Can you work these out from the model? Positions are in its coordinate system, mm. A direction names the side the tool comes from. Coordinates: 2 decimals unless noted, no trailing zeros. Order: outer loops, then holes, each group sorted by start corner. A loop starts at its lowest first (then second) coordinate and runs counter-clockwise, first axis right, second up. Notation, with made-up numbers: (14, -1.75) - (57, -1.75) arc R24 ccw to (57, 21.25) - close; hole circle Ø10 at (1, 24.5). An arc over 180 degrees is marked (long way). Return JSON: item names as keys, results as strings. Group by question number.
1) If I drill on line 1 along Z through (x, y) = (3.75, -1); line 2 along Z through (x, y) = (8.75, 1.75); line 3 along X through (y, z) = (-1.5, -2.25), over which ranges is the centre line in solid material (lowest first)?
2) Which directions (+Z, -Z, +X, -X, +Y, -Y) give clear straight access to the entire face, cutting with the end or side of a thin tool? Please do faces 4 (the face through (16, 0, 0)), 5 (the face through (0.74, 1.088, 0.616)).
3) For pin 1 Ø1 at (x, y) = (3.5, 3) entering from -Z; pin 2 Ø1.5 at (x, y) = (2.5, 0) entering from +Z; pin 3 Ø3 at (y, z) = (-1.5, 2) entering from -X; pin 4 Ø0.7 at (x, y) = (1, -0.5) entering from -Z, each with a flat end and sliding along its axis, tell me the tip position at first contact or that it passes through.
4) Imagine slicing it at A-A (x = 1.75). Write out the boundary of the cut face in (y, z), and give its area (3 significant figures).
5) Imagine slicing it at B-B (x = 14). Write out the boundary of the cut face in (y, z), and give its area (3 significant figures).
6) If we mould it in two halves opening along Z, with no side actions, what happens to faces 1 (the face through (2.106, -0.199, 0.009)), 2 (the face through (9.178, 1.847, -0.766)), 3 (the face through (0, -2, 0))? For each: pulls with the +Z half, pulls with the -Z half, needs draft (parallel to the pull), parting line crosses it, or undercut.
```python
from build123d import *

# Parameters (mm, degrees)
FILLET1_R   = 0.2
HEX_2_DEPTH = 1.5


with BuildPart() as part:
    # BodySke → BaseBody (revolve)
    with BuildSketch(Plane.XY):
        Polygon((0, 0), (0, 3.9), (0.58, 3.9), (2.48, 2), (15.61, 2), (16, 1.61), (16, 0), align=None)
    revolve(axis=Axis((0, 0, 0), (1, 0, 0)))

    # Fillet1
    fillet1_edges = [part.edges().sort_by_distance(p)[0] for p in [
        (2.48, -2, 0),
    ]]
    fillet(fillet1_edges, radius=FILLET1_R)

    # Sketch2 → PreBroach (revolve, cut)
    with BuildSketch(Plane.XY):
        Polygon((0, 1.25), (1.5, 1.25), (2.221687836, 0), (0, 0), align=None)
    revolve(axis=Axis((0, 0, 0), (1, 0, 0)), mode=Mode.SUBTRACT)

    # Sketch3 → Hex 2 (cut)
    with BuildSketch(Plane.ZY):
        Polygon((-1.25, -0.721687836), (-1.25, 0.721687836), (0, 1.443375673), (1.25, 0.721687836), (1.25, -0.721687836), (0, -1.443375673), align=None)
    extrude(amount=-HEX_2_DEPTH, mode=Mode.SUBTRACT)


solid = part.part
```
Calculated:
{
 "1": {"line 1": "-1.73 to 1.73", "line 2": "-0.97 to 0.97", "line 3": "0 to 1.78"},
 "2": {"face 4": "+Z, -Z, +X, +Y, -Y", "face 5": "-X"},
 "3": {"pin 1": "through", "pin 2": "z = 2.73", "pin 3": "x = 0", "pin 4": "z = -3.8"},
 "4": {"outline": "circle Ø5.46 at (0, 0); hole circle Ø1.63 at (0, 0)", "area": "21.3 mm2"},
 "5": {"outline": "circle Ø4 at (0, 0)", "area": "12.6 mm2"},
 "6": {"face 1": "undercut", "face 2": "parting line crosses it", "face 3": "needs draft"}
}
